Check sheet for the modelled part. Datum: model origin and axes. Units: mm. A direction names the side the tool comes from. Round coordinates to 2 decimals unless told otherwise and drop trailing zeros. Loops run counter-clockwise (first coordinate to the right, second up) from the corner with the lowest first, then second, coordinate; pieces in that order, holes last. Notation, with made-up numbers: (-6.5, -9.5) -> (19.5, -9.5) arc R8 ccw to (19.5, -1.5) -> close; hole circle Ø1 at (-37.75, 19). An arc over 180 degrees is marked (long way). One line per question, with ' | ' between items.
Autodesk Inventor part; units mm, degrees
ref_plane "YZ Plane" through (0, 0, 0) normal (1, 0, 0) x (0, 1, 0)
ref_plane "XZ Plane" through (0, 0, 0) normal (0, 1, 0) x (-1, 0, 0)
ref_plane "XY Plane" through (0, 0, 0) normal (0, 0, 1) x (1, 0, 0)
sketch "Sketch1" plane through (0, 0, 0) normal (0, 1, 0) x (-1, 0, 0)
  circle A0 centre (0, 0) radius 9.45
  circle A1 centre (0, 0) radius 8.45
  line L0 (15.45, 25) -> (15.45, -25)
  line L1 (-20, 0) -> (-15, 0)
  line L2 (-15, 0) -> (-15, 25)
  line L3 (-15, 25) -> (-20, 25)
  line L4 (-20, 25) -> (-20, 0)
  line L5 (-20, 0) -> (-15, 0)
  line L6 (-15, 0) -> (-15, -25)
  line L7 (-15, -25) -> (-20, -25)
  line L8 (-20, -25) -> (-20, 0)
  line L9 (15.45, 25) -> (-20, 25)
  line L10 (-20, 25) -> (-20, -25)
  line L11 (-20, -25) -> (15.45, -25)
  line L12 (15.45, -25) -> (15.45, 25)
  point P0 (15.45, 0)
  dimension "d0" = 18.9
  dimension "d1" = 16.9
  dimension "d7" = 5
  dimension "d8" = 20
extrude "Extrusion1" add sketch "Sketch1" along normal blind 10 contours L0 L11 L6 L2 L9 | L2 L1 L4 L3 | L7 L8 L1 L6
extrude "Extrusion2" add sketch "Sketch1" along normal blind 4.9 contours A0
sketch "Sketch2" plane through (0, 10, 0) normal (0, 1, 0) x (1, 0, 0)
  circle A0 centre (0, 0) radius 11.9
  line L0 (-15.45, -25) -> (20, -25)
  line L1 (20, 25) -> (-15.45, 25)
  line L2 (20, -25) -> (15, -25)
  line L3 (15, -25) -> (15, 25)
  line L4 (15, 25) -> (20, 25)
  line L5 (20, 25) -> (20, -25)
  line L6 (-15.45, 25) -> (-15.45, -25)
  line L7 (20, -25) -> (-15.45, -25)
  line L8 (-15.45, -25) -> (-15.45, 25)
  line L9 (-15.45, 25) -> (20, 25)
  line L10 (20, 25) -> (20, -25)
  point P0 (-6.8165, -9.7543)
  point P1 (-6.8165, 9.7543)
  dimension "d13" = 23.8
  dimension "d14" = 5
sketch "Sketch7" plane through (20, 0, -25) normal (0, 0, -1) x (-1, 0, 0)
  line L0 (35.45, 0) -> (35.45, 10)
  line L1 (0, 0) -> (35.45, 0)
  line L2 (35.45, 0) -> (35.45, 10)
  line L3 (35.45, 10) -> (0, 10)
  line L4 (0, 10) -> (0, 0)
  point P0 (20, 0)
extrude "Extrusion7" add sketch "Sketch7" along normal blind 10
sketch "Sketch8" plane through (-15.45, 0, 25) normal (0, 0, 1) x (1, 0, 0)
  line L0 (35.45, 0) -> (35.45, 10)
  line L1 (0, 0) -> (0, 10)
  line L2 (35.45, 0) -> (0, 0)
  line L3 (0, 0) -> (0, 10)
  line L4 (0, 10) -> (35.45, 10)
  line L5 (35.45, 10) -> (35.45, 0)
  point P0 (15.45, 0)
extrude "Extrusion8" add sketch "Sketch8" along normal blind 10
sketch "Sketch9" plane through (0, 10, 0) normal (0, 1, 0) x (1, 0, 0)
  circle A0 centre (0, 0) radius 11.9
  line L0 (15, -25) -> (15, 25)
  line L1 (15, -25) -> (-6.8165, -9.7543)
  line L2 (15, 25) -> (-6.8165, 9.7543)
  line L3 (20, 35) -> (20, -35)
  line L4 (20, 25) -> (15, 25)
  line L5 (15, 25) -> (15, 35)
  line L6 (15, 35) -> (20, 35)
  line L7 (20, 35) -> (20, 25)
  line L8 (20, -25) -> (15, -25)
  line L9 (15, -25) -> (15, -35)
  line L10 (15, -35) -> (20, -35)
  line L11 (20, -35) -> (20, -25)
  line L12 (15, -25) -> (15, 25)
  line L13 (-15.45, -35) -> (-15.45, 35)
  line L14 (-15.45, 25) -> (15, 25)
  line L15 (15, -25) -> (-15.45, -25)
  line L16 (-15.45, -25) -> (-15.45, 25)
  line L17 (15, -25) -> (-15.45, -25)
  line L18 (-15.45, -25) -> (-15.45, -35)
  line L19 (-15.45, -35) -> (15, -35)
  line L20 (15, -35) -> (15, -25)
  line L21 (20, 35) -> (-15.45, 35)
  line L22 (15, 25) -> (-15.45, 25)
  line L23 (-15.45, 25) -> (-15.45, 35)
  line L24 (-15.45, 35) -> (15, 35)
  line L25 (15, 35) -> (15, 25)
  point P0 (15, 25)
  dimension "d27" = 10
extrude "Extrusion9" cut sketch "Sketch9" against normal blind 10 contours A0 L1 L15 L13 L14 L2
extrude "Extrusion10" cut sketch "Sketch9" against normal blind 10 contours L14 L13 L21 L5 | L9 L19 L13 L15
fillet "Fillet1" radius 5 2 edges at (15, 5, 25) (15, 5, -25)
sketch "Sketch10" plane through (-15.45, 0, 35) normal (0, 0, 1) x (1, 0, 0)
  line L0 (35.45, 10) -> (35.45, 0)
  line L1 (30.45, 10) -> (30.45, 0)
  line L2 (35.45, 0) -> (30.45, 0)
  line L3 (30.45, 0) -> (30.45, 10)
  line L4 (30.45, 10) -> (35.45, 10)
  line L5 (35.45, 10) -> (35.45, 0)
  point P0 (15.45, 0)
extrude "Extrusion11" add sketch "Sketch10" along normal blind 2.606
sketch "Sketch11" plane through (20, 0, -35) normal (0, 0, -1) x (-1, 0, 0)
  line L0 (5, 10) -> (0, 10)
  line L1 (5, 10) -> (5, 0)
  line L2 (0, 10) -> (5, 10)
  line L3 (5, 10) -> (5, 0)
  line L4 (5, 0) -> (0, 0)
  line L5 (0, 0) -> (0, 10)
  point P0 (20, 0)
extrude "Extrusion12" add sketch "Sketch11" along normal blind 2.606
sketch "Sketch14" plane through (0, 10, 0) normal (0, 1, 0) x (1, 0, 0)
  circle A0 centre (0, 0) radius 9.45
  line L0 (15, 37.606) -> (15, 27.6058)
  arc A1 (12.8641, 23.5074) -> (15, 27.6058) centre (10, 27.6058) ccw
  line L1 (12.8641, 23.5074) -> (-6.8165, 9.7543)
  arc A2 (-6.8165, 9.7543) -> (-6.8165, -9.7543) centre (0, 0) ccw
  line L2 (-6.8165, -9.7543) -> (12.8641, -23.5074)
  arc A3 (15, -27.6058) -> (12.8641, -23.5074) centre (10, -27.6058) ccw
  line L3 (15, -27.6058) -> (15, -37.606)
  line L4 (20, -37.606) -> (15, -37.606)
  line L5 (20, 37.606) -> (20, -37.606)
  line L6 (15, 37.606) -> (20, 37.606)
extrude "Extrusion15" add sketch "Sketch14" along normal blind 2
sketch "Sketch15" plane through (0, 0, 0) normal (0, -1, 0) x (1, 0, 0)
  line L0 (15, -27.6058) -> (15, -37.606)
  line L1 (20, -37.606) -> (15, -37.606)
  line L2 (20, 37.606) -> (20, -37.606)
  line L3 (15, 37.606) -> (20, 37.606)
  line L4 (15, 37.606) -> (15, 27.6058)
  arc A0 (12.8641, 23.5074) -> (15, 27.6058) centre (10, 27.6058) ccw
  line L5 (12.8641, 23.5074) -> (-6.8165, 9.7543)
  arc A1 (-6.8165, 9.7543) -> (-6.8165, -9.7543) centre (0, 0) ccw
  line L6 (-6.8165, -9.7543) -> (12.8641, -23.5074)
  arc A2 (15, -27.6058) -> (12.8641, -23.5074) centre (10, -27.6058) ccw
  circle A3 centre (0, 0) radius 8.45
extrude "Extrusion16" add sketch "Sketch15" along normal blind 2
sketch "Sketch16" plane through (0, 4.9, 0) normal (0, 1, 0) x (1, 0, 0)
  circle A0 centre (0, 0) radius 9.45
  circle A1 centre (0, 0) radius 8.45
extrude "Extrusion17" add sketch "Sketch16" along normal blind 2.1
sketch "Sketch17" plane through (-15.45, 0, 37.606) normal (0, 0, 1) x (1, 0, 0)
  line L0 (35.45, 12) -> (35.45, -2)
  line L1 (30.45, 12) -> (35.45, 12)
  line L2 (30.45, -2) -> (30.45, 12)
  line L3 (35.45, -2) -> (30.45, -2)
  point P0 (15.45, 0)
extrude "Extrusion18" add sketch "Sketch17" along normal blind 4
sketch "Sketch18" plane through (20, 0, -37.606) normal (0, 0, -1) x (-1, 0, 0)
  line L0 (5, 12) -> (5, -2)
  line L1 (0, 12) -> (5, 12)
  line L2 (0, -2) -> (0, 12)
  line L3 (5, -2) -> (0, -2)
  point P0 (20, 0)
extrude "Extrusion19" add sketch "Sketch18" along normal blind 4
sketch "Sketch22" plane through (0, -2, 0) normal (0, -1, 0) x (1, 0, 0)
  arc A0 (-6.8165, 9.7543) -> (-6.8165, -9.7543) centre (0, 0) ccw
  line L0 (-6.8165, -9.7543) -> (12.8641, -23.5074)
  arc A1 (15, -27.6058) -> (12.8641, -23.5074) centre (10, -27.6058) ccw
  line L1 (15, -27.6058) -> (15, -41.606)
  line L2 (20, -41.606) -> (15, -41.606)
  line L3 (20, 41.606) -> (20, -41.606)
  line L4 (15, 41.606) -> (20, 41.606)
  line L5 (15, 27.6058) -> (15, 41.606)
  arc A2 (12.8641, 23.5074) -> (15, 27.6058) centre (10, 27.6058) ccw
  line L6 (12.8641, 23.5074) -> (-6.8165, 9.7543)
  circle A3 centre (0, 0) radius 8.45
extrude "Extrusion22" add sketch "Sketch22" along normal blind 1
sketch "Sketch23" plane through (-15.45, 0, 41.606) normal (0, 0, 1) x (1, 0, 0)
  line L0 (30.45, 12) -> (30.45, -3)
  line L1 (35.45, -3) -> (30.45, -3)
  line L2 (35.45, 12) -> (35.45, -3)
  line L3 (35.45, 12) -> (30.45, 12)
  line L4 (35.45, 12) -> (35.45, -3)
  line L5 (30.45, -3) -> (35.45, -3)
  line L6 (30.45, 12) -> (30.45, -3)
  line L7 (30.45, 12) -> (35.45, 12)
  point P0 (15.45, 0)
sketch "Sketch24" plane through (-15.45, 0, 41.606) normal (0, 0, 1) x (1, 0, 0)
  point P0 (15.45, 0)
extrude "Extrusion23" add sketch "Sketch23" along normal blind 1
sketch "Sketch25" plane through (20, 0, -41.606) normal (0, 0, -1) x (-1, 0, 0)
  line L0 (0, 12) -> (0, -3)
  line L1 (5, -3) -> (0, -3)
  line L2 (5, 12) -> (5, -3)
  line L3 (5, 12) -> (0, 12)
  point P0 (20, 0)
extrude "Extrusion24" add sketch "Sketch25" along normal blind 1
sketch "Sketch26" plane through (15, -3, 27.6058) normal (-1, 0, 0) x (0, 0, 1)
  line L0 (0, 0) -> (0, 15)
  line L1 (0, 0) -> (15.0002, 0)
  line L2 (15.0002, 15) -> (15.0002, 0)
  line L3 (0, 15) -> (15.0002, 15)
  circle A0 centre (7.5001, 7.5) radius 2.5
  point P0 (-27.6058, 3)
  dimension "d67" = 5
extrude "Extrusion25" cut sketch "Sketch26" against normal up to surface (5 mm away) contours A0
sketch "Sketch27" plane through (15, -3, -27.6058) normal (-1, 0, 0) x (0, 0, 1)
  line L0 (0, 15) -> (0, 0)
  line L1 (0, 15) -> (-15.0002, 15)
  line L2 (-15.0002, 0) -> (-15.0002, 15)
  line L3 (0, 0) -> (-15.0002, 0)
  circle A0 centre (-7.5001, 7.5) radius 2.5
  point P0 (27.6058, 3)
  dimension "d70" = 5
extrude "Extrusion26" cut sketch "Sketch27" against normal up to surface (5 mm away) contours A0
fillet "Fillet4" radius 3 4 edges at (17.5, 12, 42.606) (17.5, -3, 42.606) (17.5, -3, -42.606) (17.5, 12, -42.606)
sketch "Sketch28" plane through (20, 0, 42.606) normal (1, 0, 0) x (0, 0, -1)
  arc A0 (85.212, 9) -> (82.212, 12) centre (82.212, 9) ccw
  line L0 (82.212, 12) -> (3, 12)
  arc A1 (3, 12) -> (0, 9) centre (3, 9) ccw
  line L1 (0, 0) -> (0, 9)
  arc A2 (0, 0) -> (3, -3) centre (3, 0) ccw
  line L2 (3, -3) -> (82.212, -3)
  arc A3 (82.212, -3) -> (85.212, 0) centre (82.212, 0) ccw
  line L3 (85.212, 9) -> (85.212, 0)
  circle A4 centre (77.7119, 4.5) radius 2.5
  circle A5 centre (7.5001, 4.5) radius 2.5
  point P0 (42.606, 0)
extrude "Extrusion27" add sketch "Sketch28" along normal blind 3
sketch "Sketch29" plane through (0, 12, 0) normal (0, 1, 0) x (1, 0, 0)
  line L0 (15, 39.606) -> (23, 39.606)
  line L1 (15, 27.6058) -> (15, 39.606)
  arc A0 (12.8641, 23.5074) -> (15, 27.6058) centre (10, 27.6058) ccw
  line L2 (12.8641, 23.5074) -> (-6.8165, 9.7543)
  arc A1 (-6.8165, 9.7543) -> (-6.8165, -9.7543) centre (0, 0) ccw
  line L3 (-6.8165, -9.7543) -> (12.8641, -23.5074)
  arc A2 (15, -27.6058) -> (12.8641, -23.5074) centre (10, -27.6058) ccw
  line L4 (15, -27.6058) -> (15, -39.606)
  line L5 (23, -39.606) -> (15, -39.606)
  line L6 (23, 39.606) -> (23, -39.606)
  circle A3 centre (0, 0) radius 9.45
  circle A4 centre (0, 0) radius 8.45
  line L7 (15, 39.606) -> (15, 42.606)
  line L8 (15, 42.606) -> (23, 42.606)
  line L9 (23, 39.606) -> (23, 42.606)
  line L10 (15, -42.606) -> (23, -42.606)
  line L11 (15, -42.606) -> (15, -39.606)
  line L12 (23, -42.606) -> (23, -39.606)
  dimension "d76" = 18.9
  dimension "d77" = 16.9
properties part number "mancal[1]" material "Steel, Mild"
(1) Mould release check, pull along X, two halves, no side actions. Record for faces 1 (the face through (23, 5, 1)), 2 (the face through (19, 4, 42.606)), 3 (the face through (-7, 7, 5)), 4 (the face through (-11.9, 11, 0.2)): +X half, -X half, draft (parallel to the pull), parting line (faces both ways), or undercut.
Answer:
face 1: +X half | face 2: draft | face 3: undercut | face 4: -X half
(2) Go/stop test with flat-tipped pins: pin 1 (13.5 mm diameter, centred on x = 0, z = 0, fed in from -Y); pin 2 (1 mm diameter, centred on x = 10.5, y = 9, fed in from -Z); pin 3 (7.5 mm diameter, centred on y = 3, z = -35, fed in from -X); pin 4 (1.5 mm diameter, centred on x = -1.5, y = 10, fed in from -Z). Record where each tip stops, or that it passes through.
Answer:
pin 1: passes through | pin 2: stops at z = -22.2 | pin 3: stops at x = 15 | pin 4: stops at z = -13.99
(3) Sectioned sample at C-C, the plane x = 7.5. Record the cut outline in (y, z).
Answer:
outline: (-3, -19.76) -> (12, -19.76) -> (12, -5.75) -> (7, -5.75) -> (7, -3.89) -> (-3, -3.89) -> close; (-3, 3.89) -> (7, 3.89) -> (7, 5.75) -> (12, 5.75) -> (12, 19.76) -> (-3, 19.76) -> close
(4) Sectioned sample at A-A, the plane x = 16. Record the cut outline in (y, z).
Answer:
outline: (-3, -39.61) arc R3 ccw to (0, -42.61) -> (9, -42.61) arc R3 ccw to (12, -39.61) -> (12, 39.61) arc R3 ccw to (9, 42.61) -> (0, 42.61) arc R3 ccw to (-3, 39.61) -> close; hole circle Ø5 at (4.5, -35.11); hole circle Ø5 at (4.5, 35.11)
(5) Sectioned sample at B-B, the plane z = 0. Record the cut outline in (x, y), and give its area (3 significant figures).
Answer:
outline: (-11.9, -3) -> (-8.45, -3) -> (-8.45, 7) -> (-9.45, 7) -> (-9.45, 12) -> (-11.9, 12) -> (-11.9, 0) -> close; (8.45, -3) -> (23, -3) -> (23, 12) -> (9.45, 12) -> (9.45, 7) -> (8.45, 7) -> close | area: 260 mm2
(6) Set-up check for faces 5 (the face through (15, 5, 32)), 6 (the face through (19, 5, -42.606)): record each of +Z, -Z, +X, -X, +Y, -Y from which the full face is reachable in a straight line by a thin tool's end or side.
Answer:
face 5: +Z, -X, +Y, -Y | face 6: -Z, +X, -X, +Y, -Y
(7) Scan lines: probe 1 along Z at (x, y) = (20, 4.25); probe 2 along X at (y, z) = (-1.05, 0); probe 3 along X at (y, z) = (1, -28). Record each from-to range of solid material in increasing order.
Answer:
probe 1: z = -42.61 to -37.59, -32.62 to 32.62, 37.59 to 42.61 | probe 2: x = -11.9 to -8.45, 8.45 to 23 | probe 3: x = 15 to 23
(8) Sectioned sample at D-D, the plane y = 0.75. Record the cut outline in (x, z), and give its area (3 significant figures).
Answer:
outline: (-6.82, -9.75) -> (12.86, -23.51) arc R5 cw to (15, -27.61) -> (15, -42.61) -> (23, -42.61) -> (23, 42.61) -> (15, 42.61) -> (15, 27.61) arc R5 cw to (12.86, 23.51) -> (-6.82, 9.75) arc R11.9 ccw to start; hole circle Ø16.9 at (0, 0) | area: 1,290 mm2
